Work out the finished part from the listing and answer in its coordinate system (mm). Give positions to 0.01 mm unless a question says otherwise; leave off trailing zeros. Loops run counter-clockwise (first coordinate to the right, second up) from the corner with the lowest first, then second, coordinate; pieces in that order, holes last. Notation, with made-up numbers: (47, 85) - (67, 85) arc R21 cw to (67, 122) - close; hole circle Ø3 at (-37, 33.25). An arc over 180 degrees is marked (long way). Use CSV: the item, a comma, the result in double quotes.
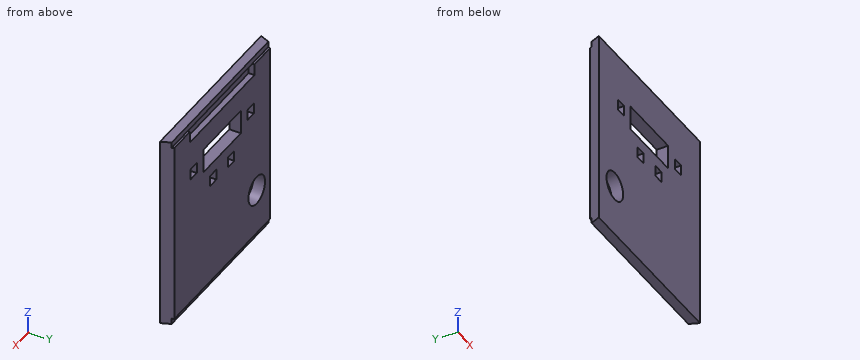
from build123d import *

# Parameters (mm, degrees)
BOSS_EXTRUDE1_DEPTH = 215.9
SKETCH2_W           = 193.548
SKETCH2_H           = 6.35
CUT_EXTRUDE1_DEPTH  = 2.3622
SKETCH3_W           = 71.628
SKETCH3_H           = 26.924
SKETCH3_W_2         = 11.938
SKETCH3_H_2         = 11.938
CUT_EXTRUDE3_DEPTH  = 291.232541773
SKETCH4_R           = 15.875
CUT_EXTRUDE4_DEPTH  = 291.232541773
CAVITY1_START       = 196.85
CAVITY1_OUTLINE_W   = 123.569632405
CAVITY1_OUTLINE_H   = 6.35
CAVITY1_DEPTH       = 12.7


# Read off the part's stored shape, not the designer's step: Cavity1
with BuildPart() as part:
    # Sketch1 → Boss-Extrude1 (new body)
    with BuildSketch(Plane.XY):
        Polygon((0, 0), (5.260512242, 12.7), (188.287487758, 12.7), (193.548, 0), align=None)
    extrude(amount=BOSS_EXTRUDE1_DEPTH)

    # Sketch2 → Cut-Extrude1 (cut)
    with BuildSketch(Plane.XZ.offset(-12.7)):
        with Locations((96.774, 3.175)):
            Rectangle(SKETCH2_W, SKETCH2_H)
        with Locations((96.774, 212.725)):
            Rectangle(SKETCH2_W, SKETCH2_H)
    extrude(amount=CUT_EXTRUDE1_DEPTH, mode=Mode.SUBTRACT)

    # Sketch3 → Cut-Extrude3 (cut, through all)
    with BuildSketch(Plane.XZ):
        with Locations((96.774, 157.988)):
            Rectangle(SKETCH3_W, SKETCH3_H)
        with Locations((79.629, 125.857)):
            Rectangle(SKETCH3_W_2, SKETCH3_H_2)
        with Locations((113.919, 125.857)):
            Rectangle(SKETCH3_W_2, SKETCH3_H_2)
        with Locations((151.257, 157.988)):
            Rectangle(SKETCH3_W_2, SKETCH3_H_2)
        with Locations((42.291, 157.988)):
            Rectangle(SKETCH3_W_2, SKETCH3_H_2)
    extrude(amount=-CUT_EXTRUDE3_DEPTH, mode=Mode.SUBTRACT)

    # Sketch4 → Cut-Extrude4 (cut, through all)
    with BuildSketch(Plane(origin=(0, 12.7, 0), x_dir=(1, 0, 0), z_dir=(0, 1, 0))):
        with Locations(Location((30.660512242, -57.15, 0), (0, 0, 180))):
            Circle(SKETCH4_R)
    extrude(amount=-CUT_EXTRUDE4_DEPTH, mode=Mode.SUBTRACT)

    # Cavity1 outline → Cavity1 (cut)
    with BuildSketch(Plane.XY.offset(CAVITY1_START)):
        with Locations((96.808185153, 9.525)):
            Rectangle(CAVITY1_OUTLINE_W, CAVITY1_OUTLINE_H)
    extrude(amount=CAVITY1_DEPTH, mode=Mode.SUBTRACT)


solid = part.part
Item 1: A cutting plane is placed at C-C on y = 3.5. Determine the outline of the cut face in (x, z) (3 decimals), and give its area (3 significant figures).
Determined:
outline,"(1.45, 0) - (192.098, 0) - (192.098, 215.9) - (1.45, 215.9) - close; hole circle Ø31.75 at (30.661, 57.15); hole (36.322, 152.019) - (48.26, 152.019) - (48.26, 163.957) - (36.322, 163.957) - close; hole (60.96, 144.526) - (132.588, 144.526) - (132.588, 171.45) - (60.96, 171.45) - close; hole (73.66, 119.888) - (85.598, 119.888) - (85.598, 131.826) - (73.66, 131.826) - close; hole (107.95, 119.888) - (119.888, 119.888) - (119.888, 131.826) - (107.95, 131.826) - close; hole (145.288, 152.019) - (157.226, 152.019) - (157.226, 163.957) - (145.288, 163.957) - close"
area,"37,900 mm²"
Item 2: A cutting plane is placed at D-D on z = 32.5. Determine the outline of the cut face in (x, y), and give its area (3 significant figures).
Determined:
outline,"(0, 0) - (193.55, 0) - (188.29, 12.7) - (5.26, 12.7) - close"
area,"2,390 mm²"
Item 3: A cutting plane is placed at B-B on x = 95.5. Determine the outline of the cut face in (y, z), and give its area (3 significant figures).
Determined:
outline,"(0, 0) - (10.34, 0) - (10.34, 6.35) - (12.7, 6.35) - (12.7, 144.53) - (0, 144.53) - close; (0, 171.45) - (12.7, 171.45) - (12.7, 196.85) - (6.35, 196.85) - (6.35, 209.55) - (10.34, 209.55) - (10.34, 215.9) - (0, 215.9) - close"
area,"2,290 mm²"
Item 4: A cutting plane is placed at A-A on z = 57.15. Determine the outline of the cut face in (x, y).
Determined:
outline,"(0, 0) - (14.79, 0) - (14.79, 12.7) - (5.26, 12.7) - close; (46.54, 0) - (193.55, 0) - (188.29, 12.7) - (46.54, 12.7) - close"
Item 5: Given P1, Ø3.5, axis at y = 5.5, z = 157, coming from the -X side; P2, Ø7, axis at y = 10.5, z = 206.5, coming from the -X side; P3, Ø3.5, axis at y = 4.5, z = 124.5, coming from the +X side, each flat-ended and moving along its own axis, determine where each tip first touches the part or whether it passes through.
Determined:
P1,"stops at x = 1.55"
P2,"stops at x = 2.9"
P3,"stops at x = 192.41"
Item 6: Find the intervals of material crossed by line 1 (Z direction, x = 99, y = 6.75); line 2 (Z direction, x = 82, y = 5.5); line 3 (Z direction, x = 117, y = 9.5), in increasing order.
Determined:
line 1,"z = 0 to 144.53, 171.45 to 196.85, 209.55 to 215.9"
line 2,"z = 0 to 119.89, 131.83 to 144.53, 171.45 to 215.9"
line 3,"z = 0 to 119.89, 131.83 to 144.53, 171.45 to 196.85, 209.55 to 215.9"
